Here's how the part is built. I have some questions about the finished solid (model axes, mm). Face numbers are marked on the shaded views. A direction names the side the tool comes from. Round coordinates to 2 decimals unless told otherwise and drop trailing zeros. Write each loop counter-clockwise with the first axis right and the second up, starting at its lowest first coordinate (ties: lowest second). Pieces come first, ordered by that corner, then holes. Notation, with made-up numbers: M 18,-16.75 L 55,-16.75 A3 cw 55,-11.75 Z; hole C -35.5,19.5 d11. An arc over 180 degrees is marked long. Write item = value, one per line. Start each with the question number.
(1) On a 3-axis mill with a long thin cutter (end or side, diameter ignored), from which of +Z, -Z, +X, -X, +Y, -Y can I reach the whole of each face in a straight line? I mean the marked faces 5 and 6. Say none if no direction works.
(2) I want a section at B-B (x = 6.3). List the corners of the cut face in (y, z) for me (3 decimals).
(3) I want a section at D-D (x = 1.5). List the corners of the cut face in (y, z) for me.
(4) I want a section at A-A (z = -6.7). List the corners of the cut face in (x, y) for me (3 decimals).
(5) If we mould it in two halves opening along X, with no side actions, what happens to the marked faces 1, 2, 3 and 4? For each: released by +X, released by -X, zero draft, split by the parting line, or undercut.
(6) Will these pins go through, and if not, where does the flat tip stop? pin 1 Ø3 at (x, z) = (7, -5.5) entering from +Y; pin 2 Ø1.5 at (x, y) = (4.5, 7.5) entering from +Z; pin 3 Ø1.5 at (y, z) = (7.5, -6) entering from +X (3 decimals); pin 4 Ø2 at (y, z) = (4, -2) entering from -X.
(7) I want a section at C-C (y = 5.25). List the corners of the cut face in (x, z) for me (3 decimals).
(8) I need wall thicknesses on line 1 along X through (y, z) = (5.9, -6.7) (3 decimals); line 2 along Z through (x, y) = (6.3, 7.1) (3 decimals); line 3 along Y through (x, z) = (11.5, -8.75). Which ranges of each line are inside material? Lowest first, please.
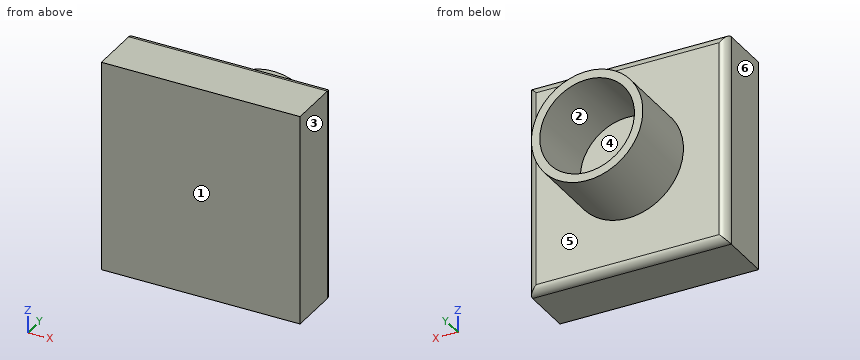
Autodesk Inventor part; units mm, degrees
ref_plane "YZ Plane" through (0, 0, 0) normal (1, 0, 0) x (0, 1, 0)
ref_plane "XZ Plane" through (0, 0, 0) normal (0, 1, 0) x (-1, 0, 0)
ref_plane "XY Plane" through (0, 0, 0) normal (0, 0, 1) x (1, 0, 0)
sketch "Sketch1" plane through (0, 0, 0) normal (0, 1, 0) x (-1, 0, 0)
  line L0 (0, 0) -> (-12.6, 0)
  line L1 (-12.6, 0) -> (-12.6, -13.4)
  line L2 (-12.6, -13.4) -> (0, -13.4)
  line L3 (0, -13.4) -> (0, 0)
  dimension "d0" = 12.6
  dimension "d1" = 13.4
extrude "Extrusion1" add sketch "Sketch1" along normal blind 3.7
sketch "Sketch2" plane through (0, 3.7, 0) normal (0, 1, 0) x (1, 0, 0)
  circle A0 centre (6.3, 6.7) radius 3.535
  line L0 (12.6, 13.4) -> (0, 13.4)
  line L1 (12.6, 0) -> (12.6, 13.4)
  circle A1 centre (6.3, 6.7) radius 3
  point P0 (0, 0)
  point P1 (6.3, 13.4)
  point P2 (12.6, 6.7)
  dimension "d4" = 7.07
  dimension "d17" = 6
extrude "Extrusion2" add sketch "Sketch2" along normal blind 4.75
fillet "Fillet1" radius 0.5 4 edges at (6.3, 3.7, 0) (12.6, 3.7, -6.7) (6.3, 3.7, -13.4) (0, 3.7, -6.7)
sketch "Sketch3" plane through (6.3, 8.45, -6.7) normal (0, 1, 0) x (1, 0, 0)
  circle A0 centre (0, 0) radius 3
  circle A1 centre (0, 0) radius 3.535
  point P0 (-6.3, -6.7)
  dimension "d7" = 6
sketch "Sketch4" plane through (6.3, 15.9, -6.7) normal (0, 1, 0) x (1, 0, 0)
  line L0 (1.46, 3.1507) -> (1.46, -2.6208)
  circle A0 centre (0, 0) radius 3 construction
  point P0 (-6.3, -6.7)
  point P1 (-3, 0)
  dimension "d13" = 4.46
properties part number "PEC12R-4017F-N0024 Base"
Returned:
q1.face_5 = +Y
q1.face_6 = +Z, -Z, -X, +Y, -Y
q2.outline = M 0,-13.4 L 3.2,-13.4 A0.5 ccw 3.7,-12.9 L 3.7,-10.235 L 8.45,-10.235 L 8.45,-9.7 L 3.7,-9.7 L 3.7,-3.7 L 8.45,-3.7 L 8.45,-3.165 L 3.7,-3.165 L 3.7,-0.5 A0.5 ccw 3.2,0 L 0,0 Z
q3.outline = M 0,-13.4 L 3.2,-13.4 A0.5 ccw 3.7,-12.9 L 3.7,-0.5 A0.5 ccw 3.2,0 L 0,0 Z
q4.outline = M 0,0 L 12.6,0 L 12.6,3.2 A0.5 ccw 12.1,3.7 L 9.835,3.7 L 9.835,8.45 L 9.3,8.45 L 9.3,3.7 L 3.3,3.7 L 3.3,8.45 L 2.765,8.45 L 2.765,3.7 L 0.5,3.7 A0.5 ccw 0,3.2 Z
q5.face_1 = zero draft
q5.face_2 = undercut
q5.face_3 = released by +X
q5.face_4 = undercut
q6.pin_1 = 3.7
q6.pin_2 = -3.32
q6.pin_3 = 9.835
q6.pin_4 = 0
q7.outline = C 6.3,-6.7 d7.07; hole C 6.3,-6.7 d6
q8.line_1 = 2.765 to 3.3, 9.3 to 9.835
q8.line_2 = -10.235 to -9.7, -3.7 to -3.165
q8.line_3 = 0 to 3.7
